Autodesk Inventor part; units mm, degrees
ref_plane "YZ Plane" through (0, 0, 0) normal (1, 0, 0) x (0, 1, 0)
ref_plane "XZ Plane" through (0, 0, 0) normal (0, 1, 0) x (-1, 0, 0)
ref_plane "XY Plane" through (0, 0, 0) normal (0, 0, 1) x (1, 0, 0)
sketch "Sketch1" plane through (0, 0, 0) normal (1, 0, 0) x (0, 1, 0)
  line L0 (3.175, 0) -> (3.175, -34.925)
  line L1 (3.175, -34.925) -> (38.1, -34.925)
  line L2 (38.1, -34.925) -> (38.1, -38.1)
  line L3 (38.1, -38.1) -> (0, -38.1)
  line L4 (0, -38.1) -> (0, 0)
  line L5 (0, 0) -> (3.175, 0)
  dimension "d0" = 3.175
  dimension "d1" = 3.175
  dimension "d2" = 38.1
  dimension "d3" = 38.1
  dimension "d4" = 0
  dimension "d5" = 0
extrude "Extrusion1" add sketch "Sketch1" along normal blind 403.225
sketch "Sketch2" plane through (0, 3.175, -34.925) normal (0, 0, 1) x (1, 0, 0)
  circle A0 centre (381.635, 13.335) radius 5.715
  line L0 (0, -3.175) -> (403.225, -3.175)
  line L1 (403.225, 34.925) -> (403.225, 0)
  line L2 (0, 0) -> (403.225, 0)
  dimension "d9" = 21.59
  dimension "d10" = 11.43
  dimension "d18" = 13.335
extrude "Extrusion2" cut sketch "Sketch2" against normal blind 25.4
sketch "Sketch3" plane through (0, 3.175, -34.925) normal (0, 0, 1) x (1, 0, 0)
  circle A0 centre (21.59, 13.335) radius 5.715
  line L0 (0, 34.925) -> (0, -3.175)
  line L1 (0, 0) -> (403.225, 0)
  dimension "d13" = 21.59
  dimension "d14" = 11.43
  dimension "d15" = 13.335
extrude "Extrusion3" cut sketch "Sketch3" against normal blind 25.4
properties part number "Side bar2"
Geometry check sheet. Reference: the model listing, model coordinates, mm. A direction names the side the tool comes from. Give positions to 0.01 mm unless a question says otherwise; leave off trailing zeros. Order: outer loops, then holes, each group sorted by start corner. A loop starts at its lowest first (then second) coordinate and runs counter-clockwise, first axis right, second up. Notation, with made-up numbers: (68, 63) - (111, 63) arc R20 ccw to (111, 77) - close; hole circle Ø9 at (75, -36.75). An arc over 180 degrees is marked (long way). Write item = value, one per line. Start each with the question number.
1) Section check A-A (x = 21.59). Enter the section's corners in (y, z) (3 decimals), then the cut area to 3 significant figures.
2) Scan lines: L1, parallel to X at y = 16, z = -36 (3 decimals); L2, parallel to Y at x = 21, z = -36; L3, parallel to Y at x = 299, z = -11.5 (3 decimals). Record each from-to range of solid material in increasing order.
3) Section check B-B (y = 16.51). Enter the section's corners in (x, z) (3 decimals).
4) Section check D-D (z = -19). Enter the section's corners in (x, y) (3 decimals), then the cut area to 3 significant figures.
5) Gauge pin test, flat ends, axial feed: pin 1 Ø7 at (x, y) = (21.59, 16.51) entering from -Z; pin 2 Ø1 at (x, z) = (120, -17) entering from +Y (3 decimals); pin 3 Ø10.5 at (x, y) = (172, 22.5) entering from +Z (3 decimals); pin 4 Ø3 at (x, z) = (111.5, -27) entering from -Y. Record the tip position at first contact, or that the pin passes through.
6) Access from +Z, -Z, +X, -X, +Y, -Y to the whole of each face (thin tool, end or side, straight path). Record for faces 5 (the flat face through (199, 3.175, -17)), 6 (the flat face through (199, 0, -19)).
7) Draft check along X on faces 1 (the cylindrical face through (24.23, 11.44, -36.49)), 2 (the flat face through (403.225, 2, -27)), 3 (the cylindrical face through (375.926, 16.761, -36.49)), 4 (the flat face through (199, 19, -38.1)). Enter one of: released by +X, released by -X, zero draft, split by the parting line, or undercut.
8) Section check C-C (x = 73). Enter the section's corners in (y, z) (3 decimals), then the cut area to 3 significant figures.
Geometry check:
q1.outline = (0, -38.1) - (10.795, -38.1) - (10.795, -34.925) - (3.175, -34.925) - (3.175, 0) - (0, 0) - close; (22.225, -38.1) - (38.1, -38.1) - (38.1, -34.925) - (22.225, -34.925) - close
q1.area = 196 mm2
q2.L1 = 0 to 15.898, 27.282 to 375.943, 387.327 to 403.225
q2.L2 = 0 to 10.83, 22.19 to 38.1
q2.L3 = 0 to 3.175
q3.outline = (0, -38.1) - (15.875, -38.1) - (15.875, -34.925) - (0, -34.925) - close; (27.305, -38.1) - (375.92, -38.1) - (375.92, -34.925) - (27.305, -34.925) - close; (387.35, -38.1) - (403.225, -38.1) - (403.225, -34.925) - (387.35, -34.925) - close
q4.outline = (0, 0) - (403.225, 0) - (403.225, 3.175) - (0, 3.175) - close
q4.area = 1,280 mm2
q5.pin_1 = through
q5.pin_2 = 3.175
q5.pin_3 = -34.925
q5.pin_4 = 0
q6.face_5 = +Z, +X, -X, +Y
q6.face_6 = +Z, -Z, +X, -X, -Y
q7.face_1 = undercut
q7.face_2 = released by +X
q7.face_3 = undercut
q7.face_4 = zero draft
q8.outline = (0, -38.1) - (38.1, -38.1) - (38.1, -34.925) - (3.175, -34.925) - (3.175, 0) - (0, 0) - close
q8.area = 232 mm2
